For this review, take the finished solid that the model builds, in its own axes (mm). A direction names the side the tool comes from. Coordinates: 2 decimals unless noted, no trailing zeros. Loops run counter-clockwise (first coordinate to the right, second up) from the corner with the lowest first, then second, coordinate; pieces in that order, holes last. Notation, with made-up numbers: M 54.5,29.5 L 84.5,29.5 A20 ccw 84.5,36.5 Z; hole C -16.75,-32.75 d1. An arc over 180 degrees is marked long. Write item = value, one per line.
Autodesk Inventor part; units mm, degrees
ref_plane "YZ Plane" through (0, 0, 0) normal (1, 0, 0) x (0, 1, 0)
ref_plane "XZ Plane" through (0, 0, 0) normal (0, 1, 0) x (-1, 0, 0)
ref_plane "XY Plane" through (0, 0, 0) normal (0, 0, 1) x (1, 0, 0)
sketch "Sketch1" plane through (0, 0, 0) normal (0, 0, 1) x (1, 0, 0)
  line L0 (0, 0) -> (230, 0)
  line L1 (230, 0) -> (230, 233.912)
  line L2 (230, 233.912) -> (0, 233.912)
  line L3 (0, 233.912) -> (0, 0)
  line L4 (38.1, 33.574) -> (191.9, 33.574)
  line L5 (191.9, 33.574) -> (191.9, 195.812)
  line L6 (191.9, 195.812) -> (38.1, 195.812)
  line L7 (38.1, 195.812) -> (38.1, 33.574)
  dimension "d0" = 230
  dimension "d1" = 233.912
  dimension "d2" = 33.574
  dimension "d3" = 38.1
  dimension "d4" = 38.1
  dimension "d5" = 38.1
extrude "Extrusion1" add sketch "Sketch1" along normal blind 6.35
fillet "Fillet3" radius 25.4 4 edges at (191.9, 33.574, 3.175) (38.1, 33.574, 3.175) (38.1, 195.812, 3.175) (191.9, 195.812, 3.175)
thicken "Thicken2" operation cut thickness 3 both sides no extend neighbours yes toward (0, 1, 0) faces at (97.8333, 195.812, 4.2333) (38.1, 96.12, 2.1167) (191.9, 133.266, 4.2333) (132.1667, 33.574, 4.2333) (183.7764, 189.0315, 2.1167) (39.8558, 179.6917, 2.1167) (180.8083, 37.9875, 2.1167) (61.6019, 33.645, 2.1167)
equation "\"d4\" = d3"
properties part number "Door Panel Front Foam" material "Polyurethane Foam"
Q1. Machinability: for faces 5 (the face through (194.9, 114, 3)), 6 (the face through (117, 233.912, 3)), which of the approach directions +Z, -Z, +X, -X, +Y, -Y give a long, thin tool a straight path to every point of the face, cutting with its end or side? Answer none if there is none.
Solved:
face_5 = +Z, -Z
face_6 = +Z, -Z, +X, -X, +Y
Q2. Add section C-C (x = 53). Write out the cut boundary in (y, z).
Solved:
outline = M 0,0 L 32.59,0 L 32.59,6.35 L 0,6.35 Z; M 196.8,0 L 233.91,0 L 233.91,6.35 L 196.8,6.35 Z
Q3. For pin 1 Ø3 at (x, z) = (130, 4) entering from -Y, flat-tipped, find the tip position at first contact; note if it passes through.
Solved:
pin_1 = 0
Q4. Add section A-A (z = 1.75). Write out the cut boundary in (x, y).
Solved:
outline = M 0,0 L 230,0 L 230,233.91 L 0,233.91 Z; hole M 35.1,58.97 A28.4 ccw 63.5,30.57 L 166.5,30.57 A28.4 ccw 194.9,58.97 L 194.9,170.41 A28.4 ccw 166.5,198.81 L 63.5,198.81 A28.4 ccw 35.1,170.41 Z
Q5. Draft analysis for pull direction X (two halves, no side actions). For faces 1 (the face through (114, 30.574, 3)), 2 (the face through (113, 0, 3)), 3 (the face through (0, 119, 3)), 4 (the face through (230, 115, 3)), state which applies: +X half, -X half, draft (parallel to the pull), parting line (faces both ways), or undercut.
Solved:
face_1 = undercut
face_2 = draft
face_3 = -X half
face_4 = +X half
Q6. Add section B-B (y = 122.5). Write out the cut boundary in (x, z).
Solved:
outline = M 0,0 L 35.1,0 L 35.1,6.35 L 0,6.35 Z; M 194.9,0 L 230,0 L 230,6.35 L 194.9,6.35 Z
Q7. For line 1 along Y through (x, z) = (109.5, 1.5); line 2 along X through (y, z) = (89, 3.75); line 3 along Y through (x, z) = (180.5, 0.75), list the stretches that pass through material, from the lowest coordinate up.
Solved:
line_1 = 0 to 30.57, 198.81 to 233.91
line_2 = 0 to 35.1, 194.9 to 230
line_3 = 0 to 34.26, 195.12 to 233.91
